from build123d import *

# Parameters (mm, degrees)
SKETCH1_W           = 50
SKETCH1_H           = 3
BOSS_EXTRUDE1_DEPTH = 10
SKETCH3_W           = 3
SKETCH3_H           = 3
CUT_EXTRUDE2_DEPTH  = 5
FILLET2_R           = 1


with BuildPart() as part:
    # Sketch1 → Boss-Extrude1 (new body)
    with BuildSketch(Plane.XY):
        with Locations((25, 1.5)):
            Rectangle(SKETCH1_W, SKETCH1_H)
    extrude(amount=BOSS_EXTRUDE1_DEPTH)

    # Sketch3 → Cut-Extrude2 (cut)
    with BuildSketch(Plane(origin=(0, 0, 0), x_dir=(-1, 0, 0), z_dir=(0, 0, -1))):
        with Locations((-81.3, 1.5)):
            Rectangle(SKETCH3_W, SKETCH3_H)
        with Locations((-60.3, 1.5)):
            Rectangle(SKETCH3_W, SKETCH3_H)
        with Locations((-40.3, 1.5)):
            Rectangle(SKETCH3_W, SKETCH3_H)
        with Locations((-24.3, 1.5)):
            Rectangle(SKETCH3_W, SKETCH3_H)
        with Locations((-6.5, 1.5)):
            Rectangle(SKETCH3_W, SKETCH3_H)
    extrude(amount=-CUT_EXTRUDE2_DEPTH, mode=Mode.SUBTRACT)

    # Fillet2
    fillet2_edges = [part.edges().sort_by_distance(p)[0] for p in [
        (38.8, 1.5, 0),
        (41.8, 1.5, 0),
        (22.8, 1.5, 0),
        (25.8, 1.5, 0),
        (5, 1.5, 0),
        (8, 1.5, 0),
    ]]
    fillet(fillet2_edges, radius=FILLET2_R)


solid = part.part
Check sheet for the modelled part. Datum: model origin and axes. Units: mm. A direction names the side the tool comes from. Round coordinates to 2 decimals unless told otherwise and drop trailing zeros. Write each loop counter-clockwise with the first axis right and the second up, starting at its lowest first coordinate (ties: lowest second). Pieces come first, ordered by that corner, then holes. Notation, with made-up numbers: (71.5, -7.75) - (80.5, -7.75) arc R22 ccw to (80.5, -0.75) - close; hole circle Ø11 at (88.25, 6). An arc over 180 degrees is marked (long way). Return JSON: item names as keys, results as strings.
Q1. Cross-section at B-B (y = 0.9). Record the boundary of the cut face in (x, z), then the cut area to 3 significant figures.
Returned:
{"outline": "(0, 0) - (4, 0) arc R1 ccw to (5, 1) - (5, 5) - (8, 5) - (8, 1) arc R1 ccw to (9, 0) - (21.8, 0) arc R1 ccw to (22.8, 1) - (22.8, 5) - (25.8, 5) - (25.8, 1) arc R1 ccw to (26.8, 0) - (37.8, 0) arc R1 ccw to (38.8, 1) - (38.8, 5) - (41.8, 5) - (41.8, 1) arc R1 ccw to (42.8, 0) - (50, 0) - (50, 10) - (0, 10) - close", "area": "454 mm²"}
Q2. Depth check by flat-ended pin: P1, Ø1.5, axis at x = 41, y = 1.5, coming from the -Z side. Enter the tip coordinate at first touch or a pass-through.
Returned:
{"P1": "stops at z = 5"}
Q3. Cross-section at C-C (x = 40). Record the boundary of the cut face in (y, z).
Returned:
{"outline": "(0, 5) - (3, 5) - (3, 10) - (0, 10) - close"}
Q4. Access from +Z, -Z, +X, -X, +Y, -Y to the whole of each face (thin tool, end or side, straight path). Record for faces 1 (the flat face through (38.8, 1, 3)), 2 (the flat face through (46, 2, 0)).
Returned:
{"face 1": "-Z, +Y, -Y", "face 2": "-Z, +X, -X, +Y, -Y"}
Q5. Scan lines: L1, parallel to X at y = 2.8, z = 3; L2, parallel to Z at x = 40, y = 1.75; L3, parallel to Z at x = 42, y = 0.55. Record each from-to range of solid material in increasing order. Write a range as from..to.
Returned:
{"L1": "x = 0..5, 8..22.8, 25.8..38.8, 41.8..50", "L2": "z = 5..10", "L3": "z = 0.4..10"}
Q6. Draft check along X on faces 3 (the flat face through (25, 2, 10)), 4 (the flat face through (0, 1, 5)), 5 (the flat face through (5, 1, 3)). Enter one of: released by +X, released by -X, zero draft, split by the parting line, or undercut.
Returned:
{"face 3": "zero draft", "face 4": "released by -X", "face 5": "undercut"}
Q7. Cross-section at A-A (z = 4.5). Record the boundary of the cut face in (x, y).
Returned:
{"outline": "(0, 0) - (5, 0) - (5, 3) - (0, 3) - close; (8, 0) - (22.8, 0) - (22.8, 3) - (8, 3) - close; (25.8, 0) - (38.8, 0) - (38.8, 3) - (25.8, 3) - close; (41.8, 0) - (50, 0) - (50, 3) - (41.8, 3) - close"}
